from build123d import *

# Parameters (mm, degrees)
SKETCH1_W           = 35
SKETCH1_H           = 35
BOSS_EXTRUDE1_DEPTH = 27
BOSS_EXTRUDE2_DEPTH = 40


with BuildPart() as part:
    # Sketch1 → Boss-Extrude1 (new body)
    with BuildSketch(Plane.XY):
        with Locations((17.5, 17.5)):
            Rectangle(SKETCH1_W, SKETCH1_H)
    extrude(amount=BOSS_EXTRUDE1_DEPTH)

    # Sketch1_3 → Boss-Extrude2 (add)
    with BuildSketch(Plane.XY):
        with BuildLine():
            ThreePointArc((19.56092483, 18.915128561), (17.5, 20), (15.43907517, 18.915128561))
            Line((15.43907517, 18.915128561), (19.56092483, 18.915128561))
        make_face()
        with BuildLine():
            Line((19.56092483, 18.915128561), (15.43907517, 18.915128561))
            ThreePointArc((15.43907517, 18.915128561), (16.759159962, 15.11229063), (20, 17.5))
            ThreePointArc((20, 17.5), (19.88770937, 18.240840038), (19.56092483, 18.915128561))
        make_face()
    extrude(amount=BOSS_EXTRUDE2_DEPTH)


solid = part.part
Geometry: final body of the model. Coordinates: model frame, mm. Give positions to 0.01 mm unless a question says otherwise; leave off trailing zeros. Write each loop counter-clockwise with the first axis right and the second up, starting at its lowest first coordinate (ties: lowest second). Pieces come first, ordered by that corner, then holes.
(1) Cut plane B-B, the plane y = 7. Return loops of the section in (x, z).
(2) First-contact query: P1, Ø5, axis at x = 21.5, y = 5.5, coming from the +Z side. Flat tip, straight axial feed; report the tip coordinate or a pass-through.
(3) Ray query, line 1 (Z direction, x = 5, y = 25.5). Return the intervals inside material, ascending.
(4) Cut plane A-A, the plane x = 17.5. Return loops of the section in (y, z), then the cut area to 3 significant figures.
Values follow:
1. outline: (0, 0) - (35, 0) - (35, 27) - (0, 27) - close
2. P1: stops at z = 27
3. line 1: z = 0 to 27
4. outline: (0, 0) - (35, 0) - (35, 27) - (20, 27) - (20, 40) - (15, 40) - (15, 27) - (0, 27) - close
4. area: 1,010 mm2
